The model under review builds one solid part; all positions refer to its coordinate system, in mm. A direction names the side the tool comes from. Coordinates: 2 decimals unless noted, no trailing zeros. Order: outer loops, then holes, each group sorted by start corner. A loop starts at its lowest first (then second) coordinate and runs counter-clockwise, first axis right, second up.
from build123d import *

# Parameters (mm, degrees)
BOSS_EXTRUDE1_DEPTH      = 30
BOSS_EXTRUDE2_DEPTH      = 5
BOSS_EXTRUDE2_DEPTH_BACK = 35
SKETCH3_R                = 3.173895943
SKETCH3_R_2              = 2.25
CUT_EXTRUDE1_DEPTH       = 15


with BuildPart() as part:
    # Sketch1 → Boss-Extrude1 (new body)
    with BuildSketch(Plane.XY):
        with BuildLine():
            Line((-45, 9.906496063), (-45, -5.093503937))
            Line((-45, -5.093503937), (-22.5, -5.093503937))
            Line((-22.5, -5.093503937), (-27.5, -0.093503937))
            Line((-27.5, -0.093503937), (27.5, -0.093503937))
            Line((27.5, -0.093503937), (22.5, -5.093503937))
            Line((22.5, -5.093503937), (45, -5.093503937))
            Line((45, -5.093503937), (45, 9.906496063))
            Line((45, 9.906496063), (35, 9.906496063))
            Line((35, 9.906496063), (35, 19.906496063))
            Line((35, 19.906496063), (25, 19.906496063))
            ThreePointArc((25, 19.906496063), (17.5, 12.406496063), (10, 19.906496063))
            Line((10, 19.906496063), (-10, 19.906496063))
            ThreePointArc((-10, 19.906496063), (-17.5, 12.406496063), (-25, 19.906496063))
            Line((-25, 19.906496063), (-35, 19.906496063))
            Line((-35, 19.906496063), (-35, 9.906496063))
            Line((-35, 9.906496063), (-45, 9.906496063))
        make_face()
    extrude(amount=BOSS_EXTRUDE1_DEPTH)

    # Sketch2 → Boss-Extrude2 (add, two sides: drawn at the far end of the back side and taken through both)
    with BuildSketch(Plane.XY.offset(30).offset(-BOSS_EXTRUDE2_DEPTH_BACK)):
        with BuildLine():
            Line((-7.5, -0.093503937), (0, 0))
            Line((0, 0), (7.5, -0.093503937))
            Line((7.5, -0.093503937), (7.5, 7.406496063))
            Line((7.5, 7.406496063), (17.5, 7.406496063))
            ThreePointArc((17.5, 7.406496063), (26.338834765, 11.067661298), (30, 19.906496063))
            Line((30, 19.906496063), (25, 19.906496063))
            ThreePointArc((25, 19.906496063), (17.5, 12.406496063), (10, 19.906496063))
            Line((10, 19.906496063), (-10, 19.906496063))
            ThreePointArc((-10, 19.906496063), (-17.5, 12.406496063), (-25, 19.906496063))
            Line((-25, 19.906496063), (-30, 19.906496063))
            ThreePointArc((-30, 19.906496063), (-26.338834765, 11.067661298), (-17.5, 7.406496063))
            Line((-17.5, 7.406496063), (-7.5, 7.406496063))
            Line((-7.5, 7.406496063), (-7.5, -0.093503937))
        make_face()
    extrude(amount=BOSS_EXTRUDE2_DEPTH + BOSS_EXTRUDE2_DEPTH_BACK)

    # Sketch3 → Cut-Extrude1 (cut)
    with BuildSketch(Plane(origin=(0, 19.906496063, 0), x_dir=(1, 0, 0), z_dir=(0, 1, 0))):
        with Locations(Location((0, 0, 0), (0, 0, 270))):
            Circle(SKETCH3_R)
        with Locations(Location((-30, -7.5, 0), (0, 0, 270))):
            Circle(SKETCH3_R_2)
        with Locations(Location((30, -7.5, 0), (0, 0, 90))):
            Circle(SKETCH3_R_2)
        with Locations(Location((30, -22.5, 0), (0, 0, 270))):
            Circle(SKETCH3_R_2)
        with Locations(Location((0, -30, 0), (0, 0, 90))):
            Circle(SKETCH3_R)
        with Locations(Location((-30, -22.5, 0), (0, 0, 90))):
            Circle(SKETCH3_R_2)
    extrude(amount=-CUT_EXTRUDE1_DEPTH, mode=Mode.SUBTRACT)


solid = part.part
(1) Insertion check: pin 1 Ø6 at (x, z) = (4.5, 2.5) entering from -Y; pin 2 Ø1.5 at (x, z) = (-11.5, -3.5) entering from -Y; pin 3 Ø1.5 at (y, z) = (2, -2.5) entering from +X. Each pin has a flat end and moves straight along its axis. Give the tip position at first contact, or say it passes through.
(2) Consider section D-D (x = 26.5). Give the boundary of the cut face in (y, z).
(3) Tool access review of faces 4 (the face through (30, 5, 30)), 5 (the face through (-30, 4.906, 23)), 6 (the face through (12, 7.406, -3)), 7 (the face through (35, 15, 15)), 8 (the face through (-35, 15, 15)): name each direction out of +Z, -Z, +X, -X, +Y, -Y from which nothing blocks a thin tool from reaching the whole face with its end or side.
(4) Wall thickness on line 1 (X direction, y = 8.5, z = 22.5); line 2 (X direction, y = 12, z = 7.5); line 3 (X direction, y = 15, z = -2): over which ranges is each line inside the solid? List them lowest first.
(5) Consider section B-B (z = 7.5). Give the boundary of the cut face in (x, y).
(6) Consider section A-A (y = 13.5). Give the number of separate pieces and of enclosed holes in the cut face, then the cut area to 3 significant figures.
(7) The part is to be moulded in two halves that separate along Z. For faces 1 (the face through (0, 10, 35)), 2 (the face through (-30, 4.906, 7)), 3 (the face through (12, 7.406, 32)), say which applies: +Z half, -Z half, draft (parallel to the pull), parting line (faces both ways), or undercut.
(8) Consider section C-C (y = 6.5). Give the boundary of the cut face in (x, z), then the cut area to 3 significant figures.
Findings:
1. pin 1: stops at y = -0.09
1. pin 2: stops at y = 7.41
1. pin 3: stops at x = 7.5
2. outline: (-5.09, 0) - (-1.09, 0) - (-1.09, 30) - (-5.09, 30) - close; (-0.09, 0) - (11.23, 0) - (11.23, -5) - (19.91, -5) - (19.91, 35) - (11.23, 35) - (11.23, 30) - (-0.09, 30) - close
3. face 4: +Z, +X, -Y
3. face 5: +Y
3. face 6: -Z, +X, -Y
3. face 7: +Z, -Z, +X, +Y
3. face 8: +Z, -Z, -X, +Y
4. line 1: x = -45 to -32.25, -27.75 to 27.75, 32.25 to 45
4. line 2: x = -35 to -32.25, -27.75 to 27.75, 32.25 to 35
4. line 3: x = -29 to -23.17, -11.83 to -2.46, 2.46 to 11.83, 23.17 to 29
5. outline: (-45, -5.09) - (-22.5, -5.09) - (-27.5, -0.09) - (27.5, -0.09) - (22.5, -5.09) - (45, -5.09) - (45, 9.91) - (35, 9.91) - (35, 19.91) - (32.25, 19.91) - (32.25, 4.91) - (27.75, 4.91) - (27.75, 19.91) - (25, 19.91) arc R7.5 cw to (10, 19.91) - (-10, 19.91) arc R7.5 cw to (-25, 19.91) - (-27.75, 19.91) - (-27.75, 4.91) - (-32.25, 4.91) - (-32.25, 19.91) - (-35, 19.91) - (-35, 9.91) - (-45, 9.91) - close
6. separate pieces: 3
6. enclosed holes: 6
6. area: 1,910 mm2
7. face 1: +Z half
7. face 2: undercut
7. face 3: draft
8. outline: (-45, 0) - (-7.5, 0) - (-7.5, -5) - (7.5, -5) - (7.5, 0) - (45, 0) - (45, 30) - (7.5, 30) - (7.5, 35) - (-7.5, 35) - (-7.5, 30) - (-45, 30) - close; hole circle Ø4.5 at (-30, 7.5); hole circle Ø4.5 at (-30, 22.5); hole circle Ø6.35 at (0, 0); hole circle Ø6.35 at (0, 30); hole circle Ø4.5 at (30, 7.5); hole circle Ø4.5 at (30, 22.5)
8. area: 2,720 mm2
